Check sheet for the drawn part. Datum: minimum x, y, z corner. Units: mm. Coordinates: 2 decimals unless noted, no trailing zeros. Loops run counter-clockwise (first coordinate to the right, second up) from the corner with the lowest first, then second, coordinate; pieces in that order, holes last. Notation, with made-up numbers: M 10.5,-17 L 20.5,-17 A16 ccw 20.5,1 Z; hole C -15,71.25 d8. An arc over 180 degrees is marked long. Answer as CSV lines item,"result". Start each with the question number.
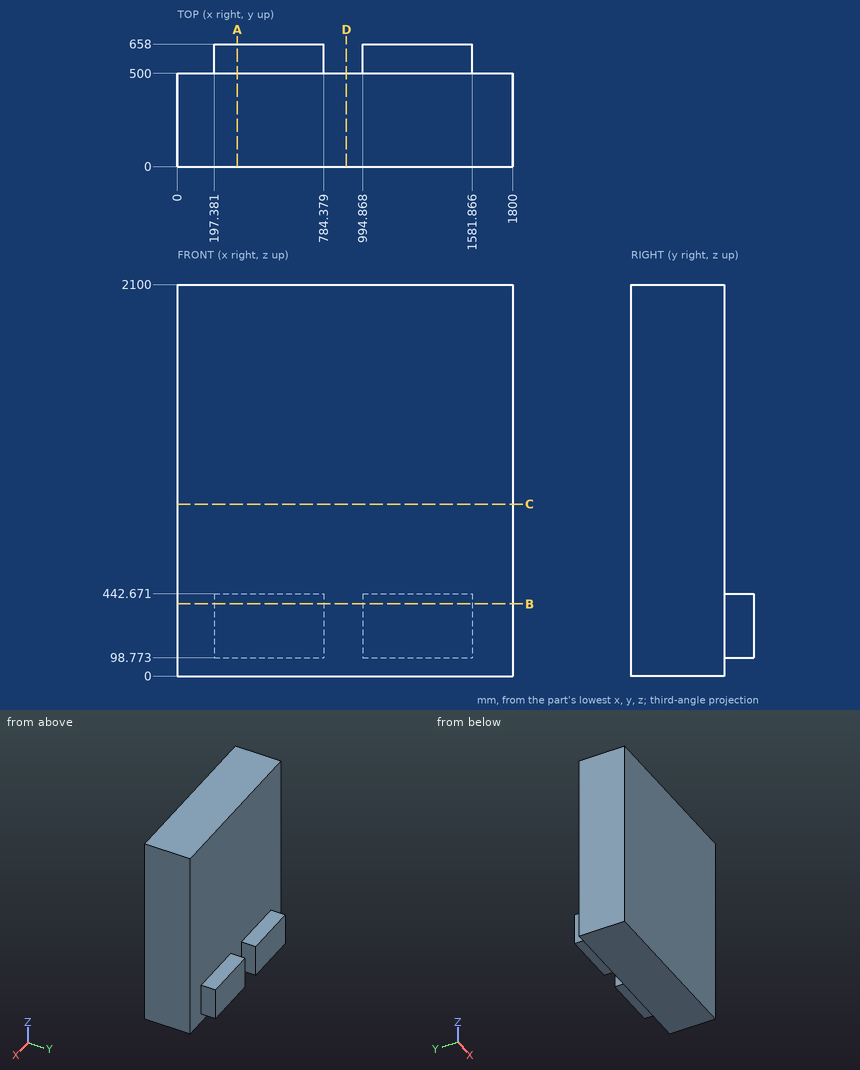
Item 1: Sectioned sample at C-C, the plane z = 922. Record the boundary of the cut face in (x, y).
Item 2: Material ranges on line 1 (Y direction, x = 1294, z = 1258); line 2 (Z direction, x = 1505.5, y = 575.5), recorded low to high. Write a range as from..to.
Item 3: Sectioned sample at D-D, the plane x = 906. Record the boundary of the cut face in (y, z).
Item 4: Go/stop test with a flat-tipped pin: pin 1 (10 mm diameter, centred on x = 469, y = 551.5, fed in from -Z). Record where the tip stops, or that it passes through.
Item 5: Sectioned sample at B-B, the plane z = 386.5. Record the boundary of the cut face in (x, y), and give its area (3 significant figures).
Item 6: Sectioned sample at A-A, the plane x = 321. Record the boundary of the cut face in (y, z), and give its area (3 significant figures).
Reply:
1,outline,"M 0,0 L 1800,0 L 1800,500 L 0,500 Z"
2,line 1,"0..500"
2,line 2,"98.77..442.67"
3,outline,"M 0,0 L 500,0 L 500,2100 L 0,2100 Z"
4,pin 1,"z = 98.77"
5,outline,"M 0,0 L 1800,0 L 1800,500 L 1581.87,500 L 1581.87,658 L 994.87,658 L 994.87,500 L 784.38,500 L 784.38,658 L 197.38,658 L 197.38,500 L 0,500 Z"
5,area,"1,090,000 mm²"
6,outline,"M 0,0 L 500,0 L 500,98.77 L 658,98.77 L 658,442.67 L 500,442.67 L 500,2100 L 0,2100 Z"
6,area,"1,100,000 mm²"
